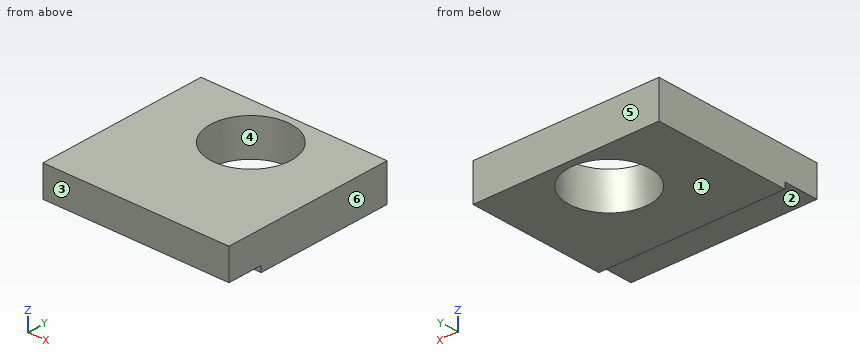
```python
from build123d import *

# Parameters (mm, degrees)
BODY_DEPTH         = 30
SKETCH_4_R         = 6.5
BEARING_HOLE_DEPTH = 6


with BuildPart() as part:
    # Эскиз1 → Body (new body)
    with BuildSketch(Plane.ZY.offset(15)):
        Polygon((137, 2.7), (137, 25), (143, 25), (143, -3), (138, -3), (138, 2.7), align=None)
    extrude(amount=-BODY_DEPTH)

    # Эскиз4 → Bearing_Hole (cut)
    with BuildSketch(Plane.XY.offset(143)):
        with Locations((0, 17.35)):
            Circle(SKETCH_4_R)
    extrude(amount=-BEARING_HOLE_DEPTH, mode=Mode.SUBTRACT)


solid = part.part
```
Source: CAD feature listing. Evaluate the final solid. Frame: model axes, mm. Face numbers are marked on the shaded views. A direction names the side the tool comes from. Give positions to 0.01 mm unless a question says otherwise; leave off trailing zeros. Order: outer loops, then holes, each group sorted by start corner. A loop starts at its lowest first (then second) coordinate and runs counter-clockwise, first axis right, second up.
(1) Section query C-C (z = 142.1). Return the cut outline in (x, y), plus the area to 3 significant figures.
(2) Access query for the marked faces 1 and 2. Directions: +Z, -Z, +X, -X, +Y, -Y. A direction counts if a zero-diameter tool reaches every point of the face in a straight line with its end or side. Return the directions, or none.
(3) Contact query for flat-ended pins moving along their axis: P1, Ø1.7, axis at x = 3.5, y = -0.5, coming from the -Z side; P2, Ø3, axis at x = -3, y = 15, coming from the -Z side. Output: stop coordinate, or through.
(4) Section query A-A (y = 17.35). Return the cut outline in (x, z), plus the area to 3 significant figures.
(5) Material intervals for line 1 along Y through (x, z) = (0, 139.1); line 2 along Z through (x, y) = (6, -1.5); line 3 along X through (y, z) = (23, 138.4), sorted ascending.
(6) Pull-direction query (Y, two-part tool) for the marked faces 3, 4, 5 and 6; classes: +Y half, -Y half, draft (parallel to the pull), parting line (faces both ways), or undercut.
(7) Section query D-D (x = -4). Return the cut outline in (y, z), plus the area to 3 significant figures.
(8) Section query B-B (x = 0). Return the cut outline in (y, z), plus the area to 3 significant figures.
Outcome:
1. outline: (-15, -3) - (15, -3) - (15, 25) - (-15, 25) - close; hole circle Ø13 at (0, 17.35)
1. area: 707 mm2
2. face 1: -Z, +X, -X, +Y, -Y
2. face 2: -Z, +X, -X, -Y
3. P1: stops at z = 138
3. P2: passes through
4. outline: (-15, 137) - (-6.5, 137) - (-6.5, 143) - (-15, 143) - close; (6.5, 137) - (15, 137) - (15, 143) - (6.5, 143) - close
4. area: 102 mm2
5. line 1: y = -3 to 10.85, 23.85 to 25
5. line 2: z = 138 to 143
5. line 3: x = -15 to -3.21, 3.21 to 15
6. face 3: -Y half
6. face 4: undercut
6. face 5: +Y half
6. face 6: draft
7. outline: (-3, 138) - (2.7, 138) - (2.7, 137) - (12.23, 137) - (12.23, 143) - (-3, 143) - close; (22.47, 137) - (25, 137) - (25, 143) - (22.47, 143) - close
7. area: 101 mm2
8. outline: (-3, 138) - (2.7, 138) - (2.7, 137) - (10.85, 137) - (10.85, 143) - (-3, 143) - close; (23.85, 137) - (25, 137) - (25, 143) - (23.85, 143) - close
8. area: 84.3 mm2
